Verification items for the finished model (mm, model axes). Face numbers are marked on the shaded views. A direction names the side the tool comes from. Give positions to 0.01 mm unless a question says otherwise; leave off trailing zeros. Write each loop counter-clockwise with the first axis right and the second up, starting at its lowest first coordinate (ties: lowest second). Pieces come first, ordered by that corner, then holes. Notation, with made-up numbers: M -9,38.5 L 45,38.5 A21 cw 45,72.5 Z; hole C 31,9 d9. An arc over 180 degrees is marked long. Write item = value, one per line.
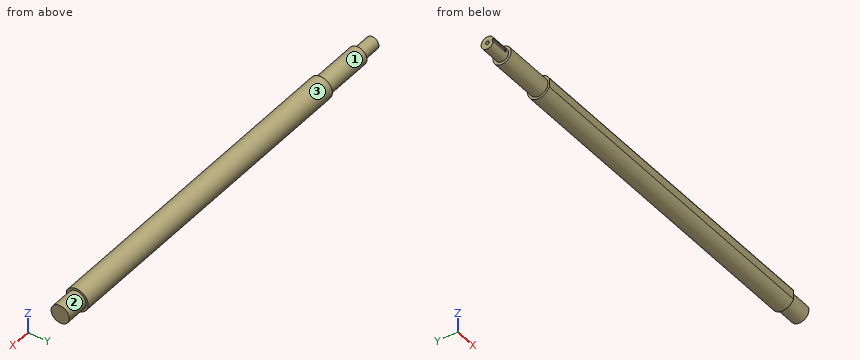
from build123d import *

# Parameters (mm, degrees)
F2_W     = 4
F2_H     = 8
F3_DEPTH = 37
F4_W     = 21.7020311332
F4_H     = 83.8147368835
F5_DEPTH = 752
F6_D     = 8
F6_DEPTH = 25
F6_TIP   = 2.4034424761


with BuildPart() as f1:
    # F0 (on Front) → F1 (revolve)
    with BuildSketch(Plane.XZ):
        Polygon((934, 0), (0, 0), (0, -14), (44, -14), (44, -20), (154, -20), (154, -25), (884, -25), (884, -20), (934, -20), align=None)
    revolve(axis=Axis((467, 0, 0), (1, 0, 0)))

    # F2 (on face) → F3 (cut)
    with BuildSketch(Plane(origin=(0, 0, 0), x_dir=(0, -1, 0), z_dir=(-1, 0, 0))):
        with Locations((13, 0)):
            Rectangle(F2_W, F2_H)
    extrude(amount=-F3_DEPTH, mode=Mode.SUBTRACT)

    # F4 (on face) → F5 (cut)
    with BuildSketch(Plane(origin=(154, 0, 0), x_dir=(0, -1, 0), z_dir=(-1, 0, 0))):
        with Locations((33.8510155666, -0.2332581207)):
            Rectangle(F4_W, F4_H)
    extrude(amount=-F5_DEPTH, mode=Mode.SUBTRACT)

    # F6
    with Locations(Plane(origin=(0, 0, 0), x_dir=(0, -1, 0), z_dir=(-1, 0, 0))):
        with Locations((0, 0)):
            Hole(F6_D / 2, depth=F6_DEPTH)
            with Locations((0, 0, -(F6_DEPTH + F6_TIP / 2))):  # 118° drill point
                Cone(0, F6_D / 2, F6_TIP, mode=Mode.SUBTRACT)


solid = f1.part
1) Cross-section at A-A on x = 723. Record the boundary of the cut face in (y, z).
From the geometry:
outline = M -23,-9.8 A25 ccw long -23,9.8 Z
2) Depth check by flat-ended pin: P1, Ø1.5, axis at y = -12, z = -1.5, coming from the -X side; P2, Ø6, axis at x = 551.5, z = 10, coming from the +Y side; P3, Ø1.9, axis at x = 20.5, y = -12, coming from the +Z side. Enter the tip coordinate at first touch or a pass-through.
From the geometry:
P1 = 37
P2 = 24
P3 = 8.6
3) Material ranges on probe 1 along Y at (x, z) = (6, 0); probe 2 along Z at (x, y) = (17, 0); probe 3 along X at (y, z) = (18, -10), recorded low to high. Write a range as from..to.
From the geometry:
probe_1 = -11..-4, 4..14
probe_2 = -14..-4, 4..14
probe_3 = 154..884
4) Cross-section at B-B on x = 118. Record the boundary of the cut face in (y, z).
From the geometry:
outline = C 0,0 d40
5) Tool access check on the marked faces 1, 2 and 3. Record the directions out of +Z, -Z, +X, -X, +Y, -Y that give a thin tool (end or side, any length) a straight path to the whole face; none if there is none.
From the geometry:
face_1 = -X
face_2 = +X
face_3 = +X, -X
